from build123d import *

# Parameters (mm, degrees)
SK_BODY_W                     = 23.65
SK_BODY_H                     = 11.1
BODY_DEPTH                    = 8.4
SK_FLANGE_EARS_W              = 4.8
SK_FLANGE_EARS_H              = 5.6
FLANGE_EARS_DEPTH             = 6
SK_NOSE_W                     = 23.65
SK_NOSE_H                     = 7
NOSE_DEPTH                    = 7.2
FLANGE_SCREW_HOLES_DEPTH      = 22.338946202
FLANGE_SCREW_HOLES_DEPTH_BACK = 22.338946202
SK_FLANGE_SCREW_HOLES_R       = 1.35
SK_WIRE_ENTRIES_W             = 2.6
SK_WIRE_ENTRIES_H             = 2.8
WIRE_ENTRIES_DEPTH            = 6
SK_CONTACT_OPENINGS_W         = 1.6
SK_CONTACT_OPENINGS_H         = 1.6
CONTACT_OPENINGS_DEPTH        = 6.2
SK_CLAMP_SCREW_HOLES_R        = 1.3
CLAMP_SCREW_HOLES_DEPTH       = 3


with BuildPart() as part:
    # SK Body → Body (new body)
    with BuildSketch(Plane.XY.offset(3)):
        with Locations((0, 1.45)):
            Rectangle(SK_BODY_W, SK_BODY_H)
    extrude(amount=BODY_DEPTH)

    # SK Flange ears → Flange ears (add)
    with BuildSketch(Plane.XY.offset(3)):
        with Locations((14.225, 0)):
            Rectangle(SK_FLANGE_EARS_W, SK_FLANGE_EARS_H)
        with Locations((-14.225, 0)):
            Rectangle(SK_FLANGE_EARS_W, SK_FLANGE_EARS_H)
    extrude(amount=FLANGE_EARS_DEPTH)

    # SK Nose → Nose (add)
    with BuildSketch(Plane.XY.offset(3)):
        with Locations((0, -0.6)):
            Rectangle(SK_NOSE_W, SK_NOSE_H)
    extrude(amount=-NOSE_DEPTH)

    # SK Flange screw holes → Flange screw holes (cut, two sides: drawn at the far end of the back side and taken through both)
    with BuildSketch(Plane.XY.offset(-FLANGE_SCREW_HOLES_DEPTH_BACK)):
        with Locations((-13.945, 0)):
            Circle(SK_FLANGE_SCREW_HOLES_R)
        with Locations((13.945, 0)):
            Circle(SK_FLANGE_SCREW_HOLES_R)
    extrude(amount=FLANGE_SCREW_HOLES_DEPTH + FLANGE_SCREW_HOLES_DEPTH_BACK, mode=Mode.SUBTRACT)

    # SK Wire entries → Wire entries (cut)
    with BuildSketch(Plane.XY.offset(11.4)):
        with Locations((-9.525, -2)):
            Rectangle(SK_WIRE_ENTRIES_W, SK_WIRE_ENTRIES_H)
        with Locations((-5.715, -2)):
            Rectangle(SK_WIRE_ENTRIES_W, SK_WIRE_ENTRIES_H)
        with Locations((-1.905, -2)):
            Rectangle(SK_WIRE_ENTRIES_W, SK_WIRE_ENTRIES_H)
        with Locations((1.905, -2)):
            Rectangle(SK_WIRE_ENTRIES_W, SK_WIRE_ENTRIES_H)
        with Locations((5.715, -2)):
            Rectangle(SK_WIRE_ENTRIES_W, SK_WIRE_ENTRIES_H)
        with Locations((9.525, -2)):
            Rectangle(SK_WIRE_ENTRIES_W, SK_WIRE_ENTRIES_H)
    extrude(amount=-WIRE_ENTRIES_DEPTH, mode=Mode.SUBTRACT)

    # SK Contact openings → Contact openings (cut)
    with BuildSketch(Plane.XY.offset(-4.2)):
        with Locations((-9.525, -0.6)):
            Rectangle(SK_CONTACT_OPENINGS_W, SK_CONTACT_OPENINGS_H)
        with Locations((-5.715, -0.6)):
            Rectangle(SK_CONTACT_OPENINGS_W, SK_CONTACT_OPENINGS_H)
        with Locations((-1.905, -0.6)):
            Rectangle(SK_CONTACT_OPENINGS_W, SK_CONTACT_OPENINGS_H)
        with Locations((1.905, -0.6)):
            Rectangle(SK_CONTACT_OPENINGS_W, SK_CONTACT_OPENINGS_H)
        with Locations((5.715, -0.6)):
            Rectangle(SK_CONTACT_OPENINGS_W, SK_CONTACT_OPENINGS_H)
        with Locations((9.525, -0.6)):
            Rectangle(SK_CONTACT_OPENINGS_W, SK_CONTACT_OPENINGS_H)
    extrude(amount=CONTACT_OPENINGS_DEPTH, mode=Mode.SUBTRACT)

    # SK Clamp screw holes → Clamp screw holes (cut)
    with BuildSketch(Plane(origin=(0, 7, 0), x_dir=(1, 0, 0), z_dir=(0, 1, 0))):
        with Locations(Location((-9.525, -7.2, 0), (0, 0, 270))):
            Circle(SK_CLAMP_SCREW_HOLES_R)
        with Locations(Location((-5.715, -7.2, 0), (0, 0, 270))):
            Circle(SK_CLAMP_SCREW_HOLES_R)
        with Locations(Location((-1.905, -7.2, 0), (0, 0, 270))):
            Circle(SK_CLAMP_SCREW_HOLES_R)
        with Locations(Location((1.905, -7.2, 0), (0, 0, 270))):
            Circle(SK_CLAMP_SCREW_HOLES_R)
        with Locations(Location((5.715, -7.2, 0), (0, 0, 270))):
            Circle(SK_CLAMP_SCREW_HOLES_R)
        with Locations(Location((9.525, -7.2, 0), (0, 0, 270))):
            Circle(SK_CLAMP_SCREW_HOLES_R)
    extrude(amount=-CLAMP_SCREW_HOLES_DEPTH, mode=Mode.SUBTRACT)


solid = part.part
Here's how the part is built. I have some questions about the finished solid (model axes, mm). A direction names the side the tool comes from. Round coordinates to 2 decimals unless told otherwise and drop trailing zeros. Write each loop counter-clockwise with the first axis right and the second up, starting at its lowest first coordinate (ties: lowest second). Pieces come first, ordered by that corner, then holes. Notation, with made-up numbers: (68, -10.75) -> (114, -10.75) arc R31 ccw to (114, 14.25) -> close; hole circle Ø5 at (87, -30.75). An arc over 180 degrees is marked (long way). One line per item, written item: value.
1) We'd pull the mould along Y, two halves only. Please class faces 6 (the face through (0, 2.9, -1)), 7 (the face through (7.015, -2, 8)), 8 (the face through (8.37, 5.52, 7.8)): released by +Y, released by -Y, zero draft, split by the parting line, or undercut.
Filled sheet:
face 6: released by +Y
face 7: undercut
face 8: zero draft
2) For faces 1 (the face through (3, 5.5, 7.9)), 2 (the face through (6, 0.2, -1)), 3 (the face through (8.225, -2, 8)), 4 (the face through (-15.294, 0.059, 5.958)), 5 (the face through (-14, 2.8, 6)), which set-ups out of +Z, -Z, +X, -X, +Y, -Y let a thin tool reach every point of the face, with its end or its side?
Filled sheet:
face 1: +Y
face 2: -Z
face 3: +Z
face 4: +Z, -Z
face 5: +Z, -Z, -X, +Y
3) Suppose I cut it at B-B on z = -2.25. List the corners of the cut face in (x, y) for me (3 decimals), plus the area to 3 significant figures.
Filled sheet:
outline: (-11.825, -4.1) -> (11.825, -4.1) -> (11.825, 2.9) -> (-11.825, 2.9) -> close; hole (-10.325, -1.4) -> (-8.725, -1.4) -> (-8.725, 0.2) -> (-10.325, 0.2) -> close; hole (-6.515, -1.4) -> (-4.915, -1.4) -> (-4.915, 0.2) -> (-6.515, 0.2) -> close; hole (-2.705, -1.4) -> (-1.105, -1.4) -> (-1.105, 0.2) -> (-2.705, 0.2) -> close; hole (1.105, -1.4) -> (2.705, -1.4) -> (2.705, 0.2) -> (1.105, 0.2) -> close; hole (4.915, -1.4) -> (6.515, -1.4) -> (6.515, 0.2) -> (4.915, 0.2) -> close; hole (8.725, -1.4) -> (10.325, -1.4) -> (10.325, 0.2) -> (8.725, 0.2) -> close
area: 150 mm2
4) Suppose I cut it at D-D on z = 7.2. Give the number of separate pieces and of enclosed holes in the cut face, plus the area to 3 significant figures.
Filled sheet:
separate pieces: 1
enclosed holes: 8
area: 214 mm2
5) Suppose I cut it at C-C on y = 3.5. List the corners of the cut face in (x, z) for me (3 decimals), plus the area to 3 significant figures.
Filled sheet:
outline: (-11.825, 3) -> (11.825, 3) -> (11.825, 11.4) -> (-11.825, 11.4) -> close
area: 199 mm2
6) Suppose I cut it at A-A on z = 10. List the corners of the cut face in (x, y) for me (3 decimals).
Filled sheet:
outline: (-11.825, -4.1) -> (11.825, -4.1) -> (11.825, 7) -> (-11.825, 7) -> close; hole (-10.825, -3.4) -> (-8.225, -3.4) -> (-8.225, -0.6) -> (-10.825, -0.6) -> close; hole (-7.015, -3.4) -> (-4.415, -3.4) -> (-4.415, -0.6) -> (-7.015, -0.6) -> close; hole (-3.205, -3.4) -> (-0.605, -3.4) -> (-0.605, -0.6) -> (-3.205, -0.6) -> close; hole (0.605, -3.4) -> (3.205, -3.4) -> (3.205, -0.6) -> (0.605, -0.6) -> close; hole (4.415, -3.4) -> (7.015, -3.4) -> (7.015, -0.6) -> (4.415, -0.6) -> close; hole (8.225, -3.4) -> (10.825, -3.4) -> (10.825, -0.6) -> (8.225, -0.6) -> close
7) I'm going to push flat-ended pins straight in: pin 1 Ø3.5 at (x, z) = (0.5, 0) entering from +Y; pin 2 Ø1.8 at (y, z) = (-0.5, -1.5) entering from -X (3 decimals); pin 3 Ø2 at (x, z) = (2, 7) entering from +Y. Where does each tip first touch, or does it pass through?
Filled sheet:
pin 1: stops at y = 2.9
pin 2: stops at x = -11.825
pin 3: stops at y = 4
8) If I drill on line 1 (X direction, y = 0, z = 5) (3 decimals); line 2 (Y direction, x = -5.5, z = 6.5); line 3 (X direction, y = 5.5, z = 4.5) (3 decimals), over which ranges is the centre line in solid material (lowest first)? Write a range as [from, to].
Filled sheet:
line 1: x = [-16.625, -15.295], [-12.595, 12.595], [15.295, 16.625]
line 2: y = [-4.1, -3.4], [-0.6, 4]
line 3: x = [-11.825, 11.825]
